from build123d import *

# Parameters (mm, degrees)
F0_W     = 20
F0_H     = 20
F1_DEPTH = 20
F2_R     = 2.6
F3_DEPTH = 1


with BuildPart() as f1:
    # F0 (on Front) → F1 (new body)
    with BuildSketch(Plane.XZ):
        with Locations((-10, 10)):
            Rectangle(F0_W, F0_H)
    extrude(amount=F1_DEPTH)

    # F2 (on face) → F3 (cut)
    with BuildSketch(Plane.XZ.offset(20)):
        with Locations((-10, 10)):
            Circle(F2_R)
        with Locations((-15, 15)):
            Circle(F2_R)
        with Locations((-5, 15)):
            Circle(F2_R)
        with Locations((-15, 5)):
            Circle(F2_R)
        with Locations((-5, 5)):
            Circle(F2_R)
    extrude(amount=-F3_DEPTH, mode=Mode.SUBTRACT)


solid = f1.part
Work out the finished part from the listing and answer in its coordinate system (mm). A direction names the side the tool comes from. Coordinates: 2 decimals unless noted, no trailing zeros. Write each loop counter-clockwise with the first axis right and the second up, starting at its lowest first coordinate (ties: lowest second). Pieces come first, ordered by that corner, then holes. Notation, with made-up numbers: (80.5, -16.5) - (107.5, -16.5) arc R21 ccw to (107.5, 2.5) - close; hole circle Ø1 at (-27, 87). An arc over 180 degrees is marked (long way). One line per question, with ' | ' between items.
1) A flat-ended cylindrical pin translates along its axis: P1, Ø1.6, axis at x = -11, z = 9.5, coming from the -Y side. Find the tip coordinate at first contact, or state that the pin passes through.
Checks:
P1: y = -19
2) For faces 1 (the face through (-3.8, -19.507, 12.693)), 2 (the face through (-10, 0, 10)), determine the directions among +Z, -Z, +X, -X, +Y, -Y from which every point of the face is accessible in a straight line to the end or side of a thin tool.
Checks:
face 1: -Y | face 2: +Z, -Z, +X, -X, +Y
3) Find section A-A, the plane z = 5. Determine the outline of the cut face in (x, y).
Checks:
outline: (-20, -20) - (-17.6, -20) - (-17.6, -19) - (-12.4, -19) - (-12.4, -20) - (-7.6, -20) - (-7.6, -19) - (-2.4, -19) - (-2.4, -20) - (0, -20) - (0, 0) - (-20, 0) - close
4) Find section B-B, the plane x = -5. Determine the outline of the cut face in (y, z).
Checks:
outline: (-20, 0) - (0, 0) - (0, 20) - (-20, 20) - (-20, 17.6) - (-19, 17.6) - (-19, 12.4) - (-20, 12.4) - (-20, 7.6) - (-19, 7.6) - (-19, 2.4) - (-20, 2.4) - close
5) The mould has two halves that part along X. Classify faces 3 (the face through (-5, -19, 5)), 4 (the face through (-8, -20, 8)), 5 (the face through (0, -10, 10)): +X half, -X half, draft (parallel to the pull), parting line (faces both ways), or undercut.
Checks:
face 3: undercut | face 4: draft | face 5: +X half
6) Consider probe 1 along Z at (x, y) = (-15, -19.8); probe 2 along Z at (x, y) = (-10, -19.4); probe 3 along Y at (x, z) = (-14, 13.5). Determine where each line is inside the solid, lowest interval first. Write a range as [from, to].
Checks:
probe 1: [0, 2.4], [7.6, 12.4], [17.6, 20] | probe 2: [0, 7.4], [12.6, 20] | probe 3: [-19, 0]
